Input: dimensioned drawing with shaded views. Units: mm. Origin: part minimum x, y, z. A direction names the side the tool comes from. Round coordinates to 2 decimals unless told otherwise and drop trailing zeros. Loops run counter-clockwise (first coordinate to the right, second up) from the corner with the lowest first, then second, coordinate; pieces in that order, holes last. Notation, with made-up numbers: (-5, 15) - (10, 15) arc R9 ccw to (10, 24) - close; hole circle Ø10 at (42.5, -7.75). An arc over 180 degrees is marked (long way). Answer as a JSON object with one key per item and string values. Group by question number.
Item 1: Section A-A (x = 10). Return the cut outline in (y, z), plus the area to 3 significant figures.
Item 2: First-contact query: pin 1 (6 mm diameter, centred on x = 10, y = 70, fed in from -Z); pin 2 (5 mm diameter, centred on y = 113, z = 8.5, fed in from +X). Flat tips, straight axial feed; report the tip coordinate or a pass-through.
Item 3: Section D-D (y = 90). Return the cut outline in (x, z), plus the area to 3 significant figures.
Item 4: Section C-C (x = 50). Return the cut outline in (y, z), plus the area to 3 significant figures.
Item 5: Line query: line 1 (Y direction, x = 50, z = 5); line 2 (Y direction, x = 52, z = 7); line 3 (Y direction, x = 9.5, z = 5). Output: solid intervals per line, ascending.
Item 6: Section B-B (y = 50). Return the cut outline in (x, z).
Item 7: Reachability of the marked faces 1 and 2 from +Z, -Z, +X, -X, +Y, -Y: full face, straight path, thin tool, end or side. Return the list, or none.
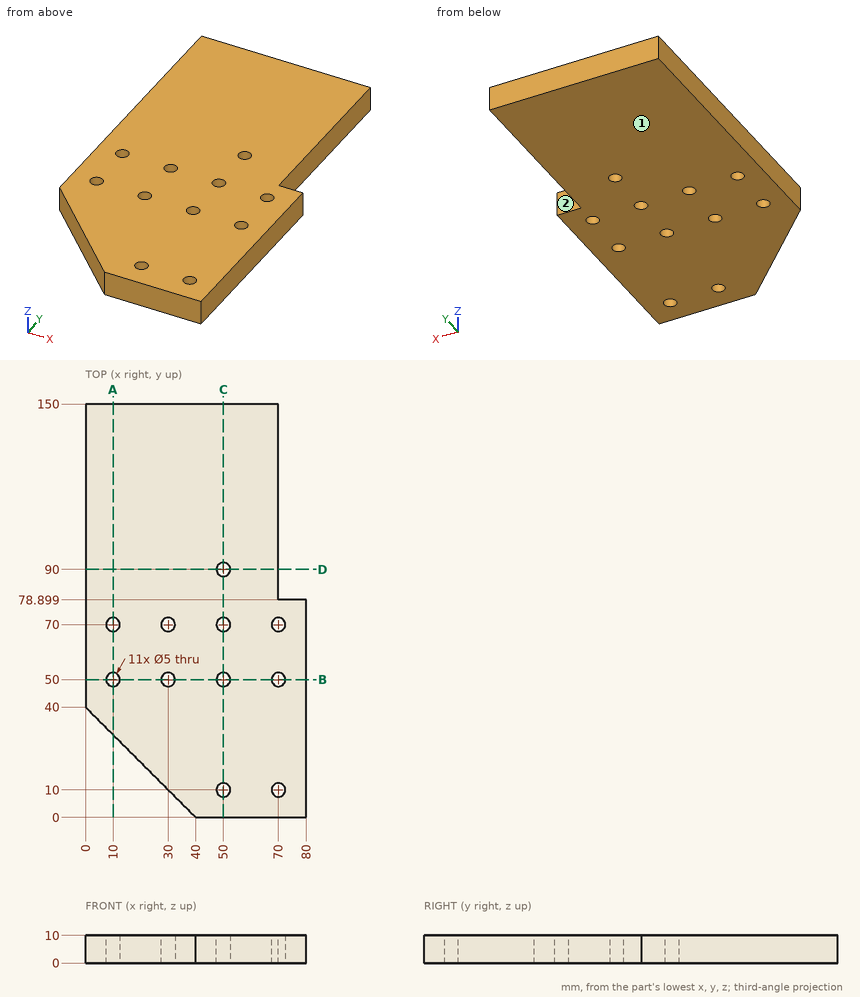
Values:
{
 "1": {"outline": "(30, 0) - (47.5, 0) - (47.5, 10) - (30, 10) - close; (52.5, 0) - (67.5, 0) - (67.5, 10) - (52.5, 10) - close; (72.5, 0) - (150, 0) - (150, 10) - (72.5, 10) - close", "area": "1,100 mm^2"},
 "2": {"pin 1": "stops at z = 0", "pin 2": "stops at x = 70"},
 "3": {"outline": "(0, 0) - (47.5, 0) - (47.5, 10) - (0, 10) - close; (52.5, 0) - (70, 0) - (70, 10) - (52.5, 10) - close", "area": "650 mm^2"},
 "4": {"outline": "(0, 0) - (7.5, 0) - (7.5, 10) - (0, 10) - close; (12.5, 0) - (47.5, 0) - (47.5, 10) - (12.5, 10) - close; (52.5, 0) - (67.5, 0) - (67.5, 10) - (52.5, 10) - close; (72.5, 0) - (87.5, 0) - (87.5, 10) - (72.5, 10) - close; (92.5, 0) - (150, 0) - (150, 10) - (92.5, 10) - close", "area": "1,300 mm^2"},
 "5": {"line 1": "y = 0 to 7.5, 12.5 to 47.5, 52.5 to 67.5, 72.5 to 87.5, 92.5 to 150", "line 2": "y = 0 to 8.5, 11.5 to 48.5, 51.5 to 68.5, 71.5 to 88.5, 91.5 to 150", "line 3": "y = 30.5 to 47.55, 52.45 to 67.55, 72.45 to 150"},
 "6": {"outline": "(0, 0) - (7.5, 0) - (7.5, 10) - (0, 10) - close; (12.5, 0) - (27.5, 0) - (27.5, 10) - (12.5, 10) - close; (32.5, 0) - (47.5, 0) - (47.5, 10) - (32.5, 10) - close; (52.5, 0) - (67.5, 0) - (67.5, 10) - (52.5, 10) - close; (72.5, 0) - (80, 0) - (80, 10) - (72.5, 10) - close"},
 "7": {"face 1": "-Z, +X, -X, +Y, -Y", "face 2": "+Z, -Z, +X, +Y"}
}
